Geometry check sheet. Reference: the model listing, model coordinates, mm. Coordinates: 2 decimals unless noted, no trailing zeros. Loops run counter-clockwise (first coordinate to the right, second up) from the corner with the lowest first, then second, coordinate; pieces in that order, holes last.
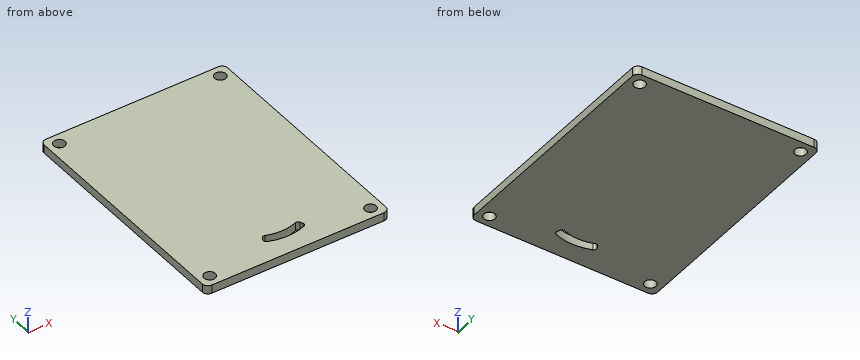
from build123d import *

# Parameters (mm, degrees)
F0_W     = 65
F0_H     = 85
F0_R     = 2
F1_DEPTH = 3
F2_R     = 2
F3_R     = 1


with BuildPart() as f1:
    # F0 (on Top) → F1 (new body)
    with BuildSketch(Plane.XY):
        with Locations((-1.109155, -6.003008)):
            Rectangle(F0_W, F0_H)
        with Locations((-29.609155, -44.503008)):
            Circle(F0_R, mode=Mode.SUBTRACT)
        with BuildLine():
            Line((-7.5, -40.125584), (-6.25, -37.398406))
            ThreePointArc((-6.25, -37.398406), (0, -38.762516), (6.25, -37.398406))
            Line((6.25, -37.398406), (7.5, -40.125584))
            ThreePointArc((7.5, -40.125584), (0, -41.762516), (-7.5, -40.125584))
        make_face(mode=Mode.SUBTRACT)
        with Locations((27.390845, -44.503008)):
            Circle(F0_R, mode=Mode.SUBTRACT)
        with Locations((-29.609155, 32.496992)):
            Circle(F0_R, mode=Mode.SUBTRACT)
        with Locations((27.390845, 32.496992)):
            Circle(F0_R, mode=Mode.SUBTRACT)
    extrude(amount=F1_DEPTH)

    # F2
    f2_edges = [f1.edges().sort_by_distance(p)[0] for p in [
        (31.390845, 36.496992, 1.5),
        (31.390845, -48.503008, 1.5),
        (-33.609155, -48.503008, 1.5),
        (-33.609155, 36.496992, 1.5),
    ]]
    fillet(f2_edges, radius=F2_R)

    # F3
    f3_edges = [f1.edges().sort_by_distance(p)[0] for p in [
        (-7.5, -40.125584, 1.5),
        (-6.25, -37.398406, 1.5),
        (6.25, -37.398406, 1.5),
        (7.5, -40.125584, 1.5),
    ]]
    fillet(f3_edges, radius=F3_R)


solid = f1.part
1) Section check B-B on z = 0.6. Record the cut outline in (x, y).
Data:
outline: (-33.61, -46.5) arc R2 ccw to (-31.61, -48.5) - (29.39, -48.5) arc R2 ccw to (31.39, -46.5) - (31.39, 34.5) arc R2 ccw to (29.39, 36.5) - (-31.61, 36.5) arc R2 ccw to (-33.61, 34.5) - close; hole circle Ø4 at (-29.61, -44.5); hole circle Ø4 at (-29.61, 32.5); hole (-7.07, -39.19) arc R1 ccw to (-6.52, -40.54) arc R18 ccw to (6.52, -40.54) arc R1 ccw to (7.07, -39.19) - (6.65, -38.28) arc R1 ccw to (5.39, -37.76) arc R15 cw to (-5.39, -37.76) arc R1 ccw to (-6.65, -38.28) - close; hole circle Ø4 at (27.39, -44.5); hole circle Ø4 at (27.39, 32.5)
2) Depth check by flat-ended pin: pin 1 (4.5 mm diameter, centred on x = 27.39, y = 32.5, fed in from -Z); pin 2 (3 mm diameter, centred on x = 27.39, y = -44.5, fed in from +Z). Enter the tip coordinate at first touch or a pass-through.
Data:
pin 1: stops at z = 0
pin 2: passes through
3) Section check A-A on x = 0. Record the cut outline in (y, z), and give its area (3 significant figures).
Data:
outline: (-48.5, 0) - (-41.76, 0) - (-41.76, 3) - (-48.5, 3) - close; (-38.76, 0) - (36.5, 0) - (36.5, 3) - (-38.76, 3) - close
area: 246 mm2
4) Material ranges on probe 1 along X at (y, z) = (32, 1.9); probe 2 along Y at (x, z) = (-28, 2.05); probe 3 along X at (y, z) = (-43.5, 0.65), recorded low to high.
Data:
probe 1: x = -33.61 to -31.55, -27.67 to 25.45, 29.33 to 31.39
probe 2: y = -48.5 to -45.69, -43.32 to 31.31, 33.68 to 36.5
probe 3: x = -33.61 to -31.34, -27.88 to 25.66, 29.12 to 31.39
5) Section check C-C on x = 27. Record the cut outline in (y, z).
Data:
outline: (-48.5, 0) - (-46.46, 0) - (-46.46, 3) - (-48.5, 3) - close; (-42.54, 0) - (30.54, 0) - (30.54, 3) - (-42.54, 3) - close; (34.46, 0) - (36.5, 0) - (36.5, 3) - (34.46, 3) - close
